from build123d import *

# Parameters (mm, degrees)
F0_W     = 100
F0_H     = 50
F1_DEPTH = 30
F2_T     = -2
F3_W     = 100
F3_H     = 2
F4_DEPTH = 10
F7_DEPTH = 2


# Not quite as in the source:
# - a pattern or mirror of a feature is missing from the dataset's text; its kind, count and spacing are read off the source's solid


with BuildPart() as f1:
    # F0 (on Top) → F1 (new body)
    with BuildSketch(Plane.XY):
        Rectangle(F0_W, F0_H)
    extrude(amount=F1_DEPTH)

    # F2
    f2_openings = [f1.faces().sort_by_distance(p)[0] for p in [
        (0, 0, 30),
    ]]
    offset(amount=F2_T, openings=f2_openings)

    # F3 (on face) → F4 (join)
    with BuildSketch(Plane(origin=(0, 25, 0), x_dir=(-1, 0, 0), z_dir=(0, 1, 0))):
        with Locations((0, 29)):
            Rectangle(F3_W, F3_H)
    f4 = extrude(amount=F4_DEPTH)

    # F4_copies: F4 across plane
    add(f4.mirror(Plane(origin=(0, 0, 0), x_dir=(0, 0, -1), z_dir=(0, -1, 0))))

    # F6 (on face) → F7 (cut, through all)
    with BuildSketch(Plane.YZ.offset(50)):
        Polygon((11.3397459622, 15), (20, 30), (-20, 30), (-11.3397459622, 15), align=None)
    extrude(amount=-F7_DEPTH, mode=Mode.SUBTRACT)


solid = f1.part
Part model, mm, in its own coordinate system. A direction names the side the tool comes from. Coordinates: 2 decimals unless noted, no trailing zeros. Loops run counter-clockwise (first coordinate to the right, second up) from the corner with the lowest first, then second, coordinate; pieces in that order, holes last. Notation, with made-up numbers: M -0.5,10 L 12.5,10 A23 cw 12.5,38 Z; hole C 37.5,59.5 d6. An arc over 180 degrees is marked long. Use a Markdown table: item, result. Add a question column.
Q1. Cut at D-D (z = 18.5). Write the cut outline in (x, y), and give its area (3 significant figures).
Q2. Mould opens along X. For faces 6 (the flat face through (-1, -25, 14)), 7 (the flat face through (-50, 0, 15)), 8 (the flat face through (-1, 23, 16)) say: +X half, -X half, draft (parallel to the pull), parting line (faces both ways), or undercut.
Q3. Cut at C-C (y = 3.5). Write the cut outline in (x, z).
Q4. Cut at B-B (x = -16.5). Write the cut outline in (y, z), and give its area (3 significant figures).
Q5. Cut at A-A (z = 9). Write the cut outline in (x, y).
Q6. Which spindle directions (+Z, -Z, +X, -X, +Y, -Y) get a long thin tool onto all of the face, cutting with end or side? Do faces 1 (the flat face through (49, 0, 15)), 2 (the flat face through (-1, 25, 14)), 3 (the flat face through (0.2, 23.5, 30)), 4 (the flat face through (-1, -23, 16)), 5 (the flat face through (1, -30, 28)). Say none if no direction does.
Q7. Pin check, flat tips, straight feed: P1, Ø1, axis at x = 17, z = 21.5, coming from the +Y side; P2, Ø1, axis at x = -32, z = 16.5, coming from the -Y side; P3, Ø5, axis at x = -24, y = 31, coming from the -Z side. Stop position of each tip, or through.
Q8. Probe L1, parallel to Y at x = -46, z = 8.5; L2, parallel to X at y = -22, z = 18.75; L3, parallel to Z at x = -7, y = 15.5. List the from-to ranges inside material, lowest first.
Worked out:
| question | item | result |
|---|---|---|
| 1 | outline | M -50,-25 L 50,-25 L 50,-13.36 L 48,-13.36 L 48,-23 L -48,-23 L -48,23 L 48,23 L 48,13.36 L 50,13.36 L 50,25 L -50,25 Z |
| 1 | area | 531 mm2 |
| 2 | face 6 | draft |
| 2 | face 7 | -X half |
| 2 | face 8 | undercut |
| 3 | outline | M -50,0 L 50,0 L 50,15 L 48,15 L 48,2 L -48,2 L -48,30 L -50,30 Z |
| 4 | outline | M -35,28 L -25,28 L -25,0 L 25,0 L 25,28 L 35,28 L 35,30 L 23,30 L 23,2 L -23,2 L -23,30 L -35,30 Z |
| 4 | area | 252 mm2 |
| 5 | outline | M -50,-25 L 50,-25 L 50,25 L -50,25 Z; hole M -48,-23 L 48,-23 L 48,23 L -48,23 Z |
| 6 | face 1 | +Z, +X |
| 6 | face 2 | -Z, +X, -X, +Y |
| 6 | face 3 | +Z, +X, -X, +Y, -Y |
| 6 | face 4 | +Z |
| 6 | face 5 | -Z, +X, -X, -Y |
| 7 | P1 | stops at y = 25 |
| 7 | P2 | stops at y = -25 |
| 7 | P3 | stops at z = 28 |
| 8 | L1 | y = -25 to -23, 23 to 25 |
| 8 | L2 | x = -50 to -48, 48 to 50 |
| 8 | L3 | z = 0 to 2 |
